```python
from build123d import *

# Parameters (mm, degrees)
SKETCH_1_R      = 8
SKETCH_1_R_2    = 2
EXTRUDE_1_DEPTH = 3
FILLET_1_R      = 10


with BuildPart() as part:
    # ｽｹｯﾁ1 → ﾎﾞｽ - 押し出し1 (new body)
    with BuildSketch(Plane.XY):
        with BuildLine():
            Line((25, -17.5), (-25, -17.5))
            Line((-25, -17.5), (-25, 17.5))
            ThreePointArc((-25, 17.5), (0, 42.5), (25, 17.5))
            Line((25, 17.5), (25, -17.5))
        make_face()
        with Locations((0, 17.5)):
            Circle(SKETCH_1_R, mode=Mode.SUBTRACT)
        with Locations((-10, -12.5)):
            Circle(SKETCH_1_R_2, mode=Mode.SUBTRACT)
        with Locations((10, -12.5)):
            Circle(SKETCH_1_R_2, mode=Mode.SUBTRACT)
    extrude(amount=EXTRUDE_1_DEPTH)

    # ﾌｨﾚｯﾄ1
    fillet_1_edges = [part.edges().sort_by_distance(p)[0] for p in [
        (25, -17.5, 1.5),
        (-25, -17.5, 1.5),
    ]]
    fillet(fillet_1_edges, radius=FILLET_1_R)


solid = part.part
```
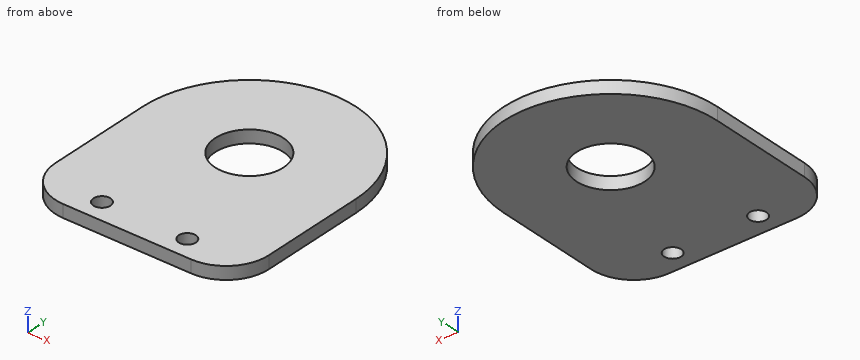
The listing builds one solid part. Answer for the finished solid, in the listing's coordinates (mm). Coordinates: 2 decimals unless noted, no trailing zeros. Loops run counter-clockwise (first coordinate to the right, second up) from the corner with the lowest first, then second, coordinate; pieces in that order, holes last. Notation, with made-up numbers: (-33.5, 55.5) - (-12.5, 55.5) arc R23 ccw to (-12.5, 74.5) - close; hole circle Ø3 at (26.25, 69.25). An arc over 180 degrees is marked (long way). Use a Markdown table: item, result. Add a question column.
1) Find the intervals of material crossed by line 1 (X direction, y = -12, z = 0.7); line 2 (Y direction, x = -4.5, z = 1.3); line 3 (Y direction, x = -2, z = 1.8), in increasing order.
2) The part is cut by section D-D, the plane y = -12.5. Give the vertices of the cut face in (x, z).
3) The part is cut by section B-B, the plane z = 1.6. Give the vertices of the cut face in (x, y), and give its area (3 significant figures).
4) The part is cut by section A-A, the plane x = 0. Give the vertices of the cut face in (y, z), and give its area (3 significant figures).
5) The part is cut by section C-C, the plane y = 23. Give the vertices of the cut face in (x, z), and give its area (3 significant figures).
Here are the results:
| question | item | result |
|---|---|---|
| 1 | line 1 | x = -23.93 to -11.94, -8.06 to 8.06, 11.94 to 23.93 |
| 1 | line 2 | y = -17.5 to 10.89, 24.11 to 42.09 |
| 1 | line 3 | y = -17.5 to 9.75, 25.25 to 42.42 |
| 2 | outline | (-23.66, 0) - (-12, 0) - (-12, 3) - (-23.66, 3) - close; (-8, 0) - (8, 0) - (8, 3) - (-8, 3) - close; (12, 0) - (23.66, 0) - (23.66, 3) - (12, 3) - close |
| 3 | outline | (-25, -7.5) arc R10 ccw to (-15, -17.5) - (15, -17.5) arc R10 ccw to (25, -7.5) - (25, 17.5) arc R25 ccw to (-25, 17.5) - close; hole circle Ø4 at (-10, -12.5); hole circle Ø16 at (0, 17.5); hole circle Ø4 at (10, -12.5) |
| 3 | area | 2,460 mm^2 |
| 4 | outline | (-17.5, 0) - (9.5, 0) - (9.5, 3) - (-17.5, 3) - close; (25.5, 0) - (42.5, 0) - (42.5, 3) - (25.5, 3) - close |
| 4 | area | 132 mm^2 |
| 5 | outline | (-24.39, 0) - (-5.81, 0) - (-5.81, 3) - (-24.39, 3) - close; (5.81, 0) - (24.39, 0) - (24.39, 3) - (5.81, 3) - close |
| 5 | area | 111 mm^2 |
